Part model, mm, in its own coordinate system. A direction names the side the tool comes from. Coordinates: 2 decimals unless noted, no trailing zeros. Write each loop counter-clockwise with the first axis right and the second up, starting at its lowest first coordinate (ties: lowest second). Pieces come first, ordered by that corner, then holes. Notation, with made-up numbers: (27.25, 61.25) - (75.25, 61.25) arc R15 ccw to (75.25, 74.25) - close; hole circle Ø2 at (-39.75, 88.25). An arc over 180 degrees is marked (long way). Use a Markdown table: item, result.
```python
from build123d import *

# Parameters (mm, degrees)
F2_SIZE        = 1
F5_DEPTH       = 5
F8_D           = 5
F8_DEPTH       = 15
F8_CSINK_D     = 13.44
F8_CSINK_ANGLE = 90
F8_TIP         = 1.5021515476


with BuildPart() as f1:
    # F0 (on Front) → F1 (revolve)
    with BuildSketch(Plane.XZ):
        Polygon((-10, -31.0083918493), (0, -31.0083918493), (0, 118.9916081507), (-20, 118.9916081507), (-20, 78.9916081507), (-25, 78.9916081507), (-25, 33.9916081507), (-10, 33.9916081507), align=None)
    revolve(axis=Axis((0, 0, 43.9916081507), (0, 0, -1)))

    # F2
    f2_edges = [f1.edges().sort_by_distance(p)[0] for p in [
        (10, 0, -31.008392),
        (25, 0, 33.991608),
        (25, 0, 78.991608),
        (20, 0, 118.991608),
    ]]
    chamfer(f2_edges, length=F2_SIZE)

    # F4 (on offset) → F5 (cut)
    with BuildSketch(Plane.YZ.offset(-10)):
        with BuildLine():
            Line((-3, -31.0083918493), (3, -31.0083918493))
            Line((3, -31.0083918493), (3, -14.0083918493))
            ThreePointArc((3, -14.0083918493), (2.1213203436, -11.8870715058), (0, -11.0083918493))
            ThreePointArc((0, -11.0083918493), (-2.1213203436, -11.8870715058), (-3, -14.0083918493))
            Line((-3, -14.0083918493), (-3, -31.0083918493))
        make_face()
    extrude(amount=F5_DEPTH, mode=Mode.SUBTRACT)

    # F8
    with Locations(Plane(origin=(0, 0, -31.0083918493), x_dir=(1, 0, 0), z_dir=(0, 0, -1))):
        with Locations((0, 0)):
            CounterSinkHole(F8_D / 2, F8_CSINK_D / 2, depth=F8_DEPTH, counter_sink_angle=F8_CSINK_ANGLE)
            with Locations((0, 0, -(F8_DEPTH + F8_TIP / 2))):  # 118° drill point
                Cone(0, F8_D / 2, F8_TIP, mode=Mode.SUBTRACT)


solid = f1.part
```
Item 1: Drop flat-ended pins along their axis: P1, Ø5, axis at x = -6, z = 26, coming from the +Y side; P2, Ø1, axis at x = -16, z = 71.5, coming from the -Y side; P3, Ø4, axis at x = -8.5, z = 86, coming from the -Y side; P4, Ø10, axis at x = 15.5, z = -14, coming from the -Y side (3 decimals). Give the stop position or say it passes through.
From the geometry:
| item | result |
|---|---|
| P1 | y = 9.37 |
| P2 | y = -19.62 |
| P3 | y = -18.91 |
| P4 | through |
Item 2: Band-saw the part on B-B, the plane z = 48. Give the cut face in (x, y), then the cut area to 3 significant figures.
From the geometry:
| item | result |
|---|---|
| outline | circle Ø50 at (0, 0) |
| area | 1,960 mm^2 |
Item 3: Band-saw the part on C-C, the plane z = 18. Give the cut face in (x, y).
From the geometry:
| item | result |
|---|---|
| outline | circle Ø20 at (0, 0) |
Item 4: Which spindle directions (+Z, -Z, +X, -X, +Y, -Y) get a long thin tool onto all of the face, cutting with end or side? Do faces 5 (the face through (-5, 20, 78.992)), 6 (the face through (-7, -3, -22)), 7 (the face through (-23.846, 7.509, 56.191)), 8 (the face through (0.54, 2.44, -21.32)), 9 (the face through (7, 1, -31.008)). Say none if no direction does.
From the geometry:
| item | result |
|---|---|
| face 5 | +Z |
| face 6 | -Z, -X |
| face 7 | +Z, -Z |
| face 8 | -Z |
| face 9 | -Z, +X, -X, +Y, -Y |
Item 5: Band-saw the part on A-A, the plane z = -20. Give the cut face in (x, y).
From the geometry:
| item | result |
|---|---|
| outline | (-9.54, -3) arc R10 ccw (long way) to (-9.54, 3) - (-5, 3) - (-5, -3) - close; hole circle Ø5 at (0, 0) |
Item 6: Two-plate mould, pull along X, no slides. Class faces 1 (the face through (2.7, -0.12, -26.99)), 2 (the face through (2.17, -9.76, 1.54)), 3 (the face through (-7, 3, -23)), 4 (the face through (-0.094, 0.424, -14.767)): pulls with the +X half, pulls with the -X half, needs draft (parallel to the pull), parting line crosses it, or undercut.
From the geometry:
| item | result |
|---|---|
| face 1 | undercut |
| face 2 | parting line crosses it |
| face 3 | needs draft |
| face 4 | undercut |
Item 7: Drill centre lines: probe 1 along Y at (x, z) = (0, -22); probe 2 along Z at (x, y) = (-16, -6); probe 3 along Z at (x, y) = (-14.5, 15.5). Where is each one in solid material? Low to high.
From the geometry:
| item | result |
|---|---|
| probe 1 | -10 to -2.5, 2.5 to 10 |
| probe 2 | 33.99 to 118.99 |
| probe 3 | 33.99 to 78.99 |
